from build123d import *

# Parameters (mm, degrees)
F0_R           = 101.673036
F1_DEPTH       = 10.16
F2_R           = 50.825474
F3_DEPTH       = 15.24
F5_D           = 50.8
F7_D           = 11.43
F7_CSINK_D     = 15.24
F7_CSINK_ANGLE = 90
F9_D           = 2.54
F10_SIZE       = 1.016


with BuildPart() as f1:
    # F0 (on Top) → F1 (new body)
    with BuildSketch(Plane.XY):
        Circle(F0_R)
    extrude(amount=F1_DEPTH)

    # F2 (on face) → F3 (join)
    with BuildSketch(Plane.XY.offset(10.16)):
        Circle(F2_R)
    extrude(amount=F3_DEPTH)

    # F5 (through all)
    with Locations(Plane.XY.offset(25.4)):
        with Locations((0, 0)):
            Hole(F5_D / 2)

    # F7 (through all)
    with Locations(Plane.XY.offset(25.4)):
        with Locations((0, 38.806446), (-36.907123, 11.991851), (-22.809857, -31.395074), (22.809857, -31.395074), (36.907123, 11.991851)):
            CounterSinkHole(F7_D / 2, F7_CSINK_D / 2, counter_sink_angle=F7_CSINK_ANGLE)

    # F9 (through all)
    with Locations(Plane.XY.offset(10.16)):
        with Locations((10.266128, 92.69405), (-46.178724, 81.025341), (-23.668928, 72.845469), (0.032693, 63.665586), (23.668928, 72.845469), (37.448142, 51.487324), (62.789668, 68.956783), (61.966057, 45.020975), (60.559673, 19.642655), (91.329689, 18.880369), (76.594258, 0), (60.539468, -19.704841), (84.984873, -38.407705), (61.966057, -45.020975), (37.395243, -51.525757), (46.178724, -81.025341), (23.668928, -72.845469), (-0.032693, -63.665586), (-10.266128, -92.69405), (-23.668928, -72.845469), (-37.448142, -51.487324), (-62.789668, -68.956783), (-61.966057, -45.020975), (-60.559673, -19.642655), (-91.329689, -18.880369), (-76.594258, 0), (-60.539468, 19.704841), (-84.984873, 38.407705), (-61.966057, 45.020975), (-37.395243, 51.525757)):
            Hole(F9_D / 2)

    # F10
    f10_edges = [f1.edges().sort_by_distance(p)[0] for p in [
        (101.673036, 0, 5.08),
        (-101.673036, 0, 0),
        (-101.673036, 0, 10.16),
    ]]
    chamfer(f10_edges, length=F10_SIZE)


solid = f1.part
The model under review builds one solid part; all positions refer to its coordinate system, in mm. A direction names the side the tool comes from. Coordinates: 2 decimals unless noted, no trailing zeros. Loops run counter-clockwise (first coordinate to the right, second up) from the corner with the lowest first, then second, coordinate; pieces in that order, holes last. Notation, with made-up numbers: M -25,83.5 L -4,83.5 A16 ccw -4,93.5 Z; hole C -24.75,64 d9. An arc over 180 degrees is marked long. Put each result on its own line as item: value. Start each with the question number.
Q1. Wall thickness on line 1 (X direction, y = 10, z = 3); line 2 (Y direction, x = 39.5, z = 17.75); line 3 (Y direction, x = 46, z = 9.5): over which ranges is each line inside the solid? List them lowest first.
Q2. For faces 5 (the cylindrical face through (5.506, -24.796, 12.522)), 6 (the flat face through (-46, 24, 10.16)), list the 3-axis set-ups (+Z, -Z, +X, -X, +Y, -Y) from which the entire face can be reached by the end or side of a thin tool; tool diameter is ignored.
Q3. The part is to be moulded in two halves that separate along X. For faces 1 (the cylindrical face through (17.36, -29.68, 11.58)), 2 (the flat face through (21, -21, 0)), 3 (the cylindrical face through (-17.1, -31.14, 11.58)), 4 (the cylindrical face through (48.478, 15.267, 17.673)), say which applies: +X half, -X half, draft (parallel to the pull), parting line (faces both ways), or undercut.
Q4. Clearance check with flat-ended pins moving along their axes: pin 1 (3.5 mm diameter, centred on x = -61.97, y = -45.02, fed in from +Z); pin 2 (2 mm diameter, centred on x = -23.67, y = 72.85, fed in from +Z); pin 3 (3 mm diameter, centred on x = 19.5, z = 4, fed in from +Y); pin 4 (15 mm diameter, centred on x = -22.81, y = -31.4, fed in from +Z). State where each tip first meets the part, or that it passes through.
Q5. Add section A-A (z = 19). Write out the cut boundary in (x, y) (3 decimals).
Answers:
1. line 1: x = -101.18 to -42.26, -31.55 to -23.35, 23.35 to 31.55, 42.26 to 101.18
1. line 2: y = -31.98 to 6.9, 17.08 to 31.98
1. line 3: y = -90.27 to -82.28, -79.77 to 90.27
2. face 5: +Z, -Z
2. face 6: +Z
3. face 1: undercut
3. face 2: draft
3. face 3: undercut
3. face 4: parting line
4. pin 1: stops at z = 10.16
4. pin 2: passes through
4. pin 3: stops at y = 100.07
4. pin 4: stops at z = 25.28
5. outline: C 0,0 d101.651; hole C -36.907,11.992 d11.43; hole C -22.81,-31.395 d11.43; hole C 0,0 d50.8; hole C 0,38.806 d11.43; hole C 22.81,-31.395 d11.43; hole C 36.907,11.992 d11.43
